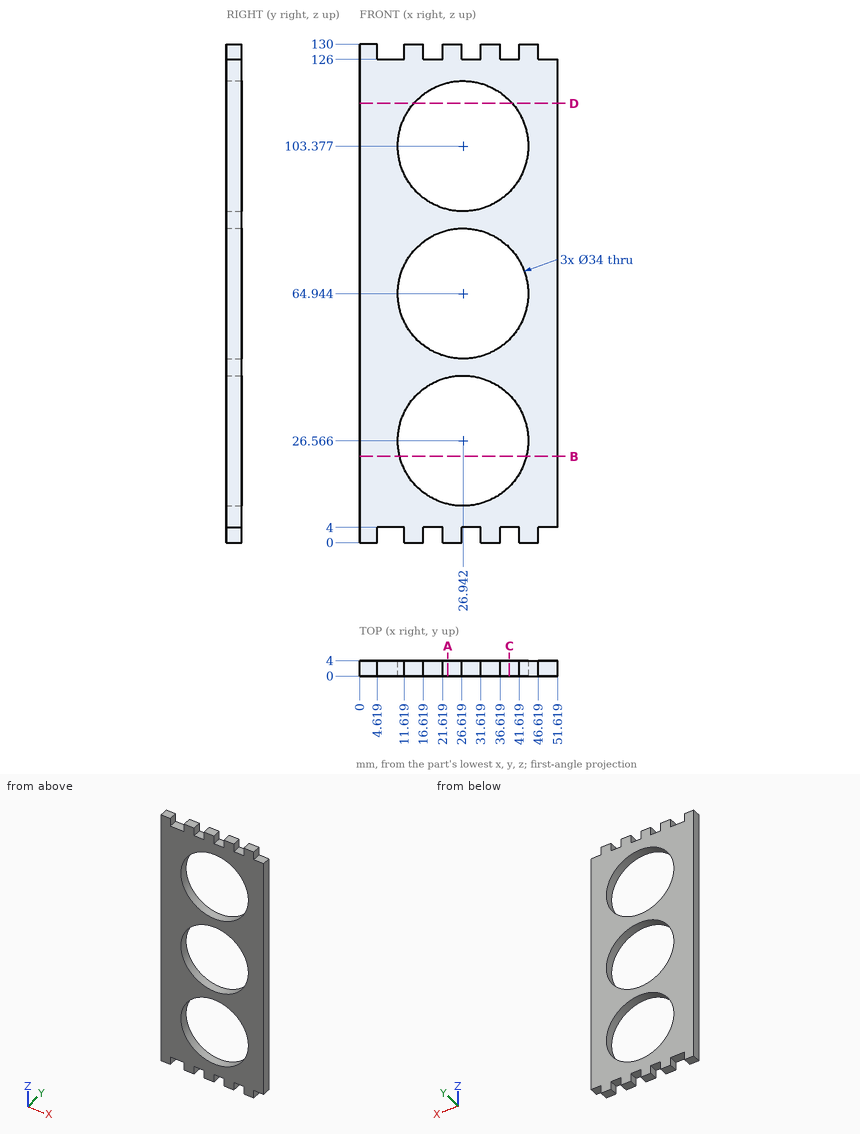
Here's the drawing with two shaded views (mm, measured from the low corner). I have some questions. Give positions to 0.01 mm unless a question says otherwise; leave off trailing zeros. Loops run counter-clockwise (first coordinate to the right, second up) from the corner with the lowest first, then second, coordinate; pieces in that order, holes last. Notation, with made-up numbers: M 19,11.25 L 56,11.25 A22 cw 56,41.25 Z; hole C 64.25,-6 d2. An arc over 180 degrees is marked long. One line per item, written item: value.
(1) Will these pins go through, and if not, where does the flat tip stop? pin 1 (1.5 mm diameter, centred on y = 2.5, z = 79, fed in from -X); pin 2 (1.2 mm diameter, centred on y = 2, z = 3, fed in from +X); pin 3 (2 mm diameter, centred on x = 48.5, y = 3, fed in from +Z); pin 4 (2 mm diameter, centred on x = 39, y = 2, fed in from -Z).
Returned:
pin 1: x = 0
pin 2: x = 46.62
pin 3: z = 126
pin 4: z = 4
(2) Suppose I cut it at D-D on z = 114.5. List the corners of the cut face in (x, y) for me (1 decimal), plus the area to 3 significant figures.
Returned:
outline: M 0,0 L 14.1,0 L 14.1,4 L 0,4 Z; M 39.8,0 L 51.6,0 L 51.6,4 L 39.8,4 Z
area: 104 mm^2
(3) Suppose I cut it at C-C on x = 39. List the corners of the cut face in (y, z) for me (1 decimal).
Returned:
outline: M 0,4 L 4,4 L 4,14.6 L 0,14.6 Z; M 0,38.5 L 4,38.5 L 4,53 L 0,53 Z; M 0,76.9 L 4,76.9 L 4,91.4 L 0,91.4 Z; M 0,115.4 L 4,115.4 L 4,126 L 0,126 Z
(4) Suppose I cut it at B-B on z = 22.5. List the corners of the cut face in (x, y) for me (1 decimal).
Returned:
outline: M 0,0 L 10.4,0 L 10.4,4 L 0,4 Z; M 43.4,0 L 51.6,0 L 51.6,4 L 43.4,4 Z
(5) I need wall thicknesses on line 1 (X direction, y = 0.85, z = 64.5) (1 decimal); line 2 (Z direction, x = 17, y = 3.7) (1 decimal); line 3 (Z direction, x = 40.5, y = 3.1) (1 decimal). Which ranges of each line are inside material? Lowest first, please.
Returned:
line 1: 0 to 9.9, 43.9 to 51.6
line 2: 4 to 12.8, 40.4 to 51.2, 78.7 to 89.6, 117.2 to 126
line 3: 4 to 16.3, 36.8 to 54.7, 75.2 to 93.1, 113.6 to 126
(6) Suppose I cut it at A-A on x = 23. List the corners of the cut face in (y, z) for me (1 decimal), plus the area to 3 significant figures.
Returned:
outline: M 0,0 L 4,0 L 4,10 L 0,10 Z; M 0,43.1 L 4,43.1 L 4,48.4 L 0,48.4 Z; M 0,81.5 L 4,81.5 L 4,86.8 L 0,86.8 Z; M 0,119.9 L 4,119.9 L 4,130 L 0,130 Z
area: 123 mm^2
